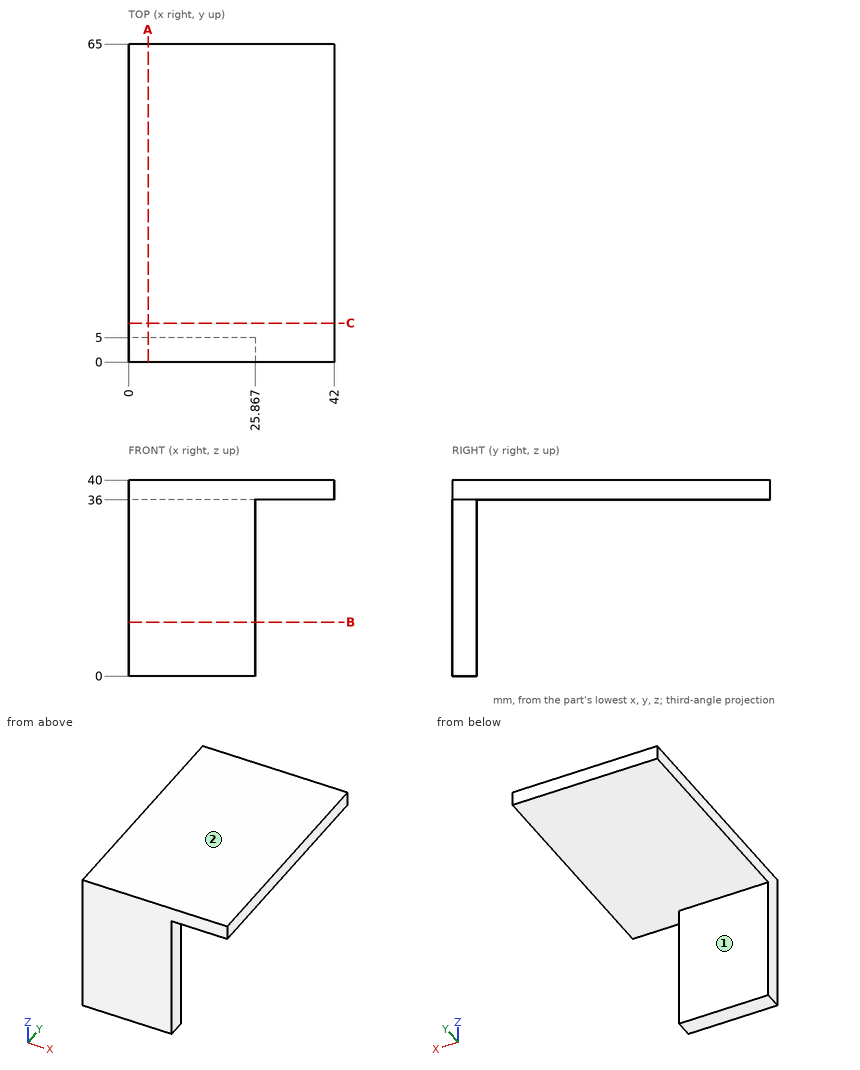
Geometry check sheet. Reference: drawing and pictorial views, mm from the part's lowest x, y, z. A direction names the side the tool comes from. Coordinates: 2 decimals unless noted, no trailing zeros. Order: outer loops, then holes, each group sorted by start corner. A loop starts at its lowest first (then second) coordinate and runs counter-clockwise, first axis right, second up.
Item 1: Section check B-B, the plane z = 11. Enter the section's corners in (x, y).
Filled in:
outline: (0, 0) - (25.87, 0) - (25.87, 5) - (0, 5) - close
Item 2: Section check C-C, the plane y = 8. Enter the section's corners in (x, z).
Filled in:
outline: (0, 36) - (42, 36) - (42, 40) - (0, 40) - close
Item 3: Section check A-A, the plane x = 4. Enter the section's corners in (y, z), then the cut area to 3 significant figures.
Filled in:
outline: (0, 0) - (5, 0) - (5, 36) - (65, 36) - (65, 40) - (0, 40) - close
area: 440 mm2
Item 4: Depth check by flat-ended pin: pin 1 (20.5 mm diameter, centred on x = 15.5, z = 14.5, fed in from +Y); pin 2 (2.5 mm diameter, centred on y = 1.5, z = 17.5, fed in from +X); pin 3 (2 mm diameter, centred on x = 15, y = 49.5, fed in from -Z); pin 4 (8 mm diameter, centred on y = 12.5, z = 10, fed in from +X). Enter the tip coordinate at first touch or a pass-through.
Filled in:
pin 1: stops at y = 5
pin 2: stops at x = 25.87
pin 3: stops at z = 36
pin 4: passes through
Item 5: Access from +Z, -Z, +X, -X, +Y, -Y to the whole of each face (thin tool, end or side, straight path). Record for the marked faces 1 and 2.
Filled in:
face 1: -Z, +X, -X, +Y
face 2: +Z, +X, -X, +Y, -Y
Item 6: Material ranges on L1, parallel to Z at x = 28, y = 40; L2, parallel to Y at x = 13, z = 15; L3, parallel to X at y = 4.5, z = 5, recorded low to high.
Filled in:
L1: z = 36 to 40
L2: y = 0 to 5
L3: x = 0 to 25.87
